Geometry: final body of the model. Coordinates: model frame, mm. A direction names the side the tool comes from. Give positions to 0.01 mm unless a question says otherwise; leave off trailing zeros. Write each loop counter-clockwise with the first axis right and the second up, starting at its lowest first coordinate (ties: lowest second). Pieces come first, ordered by that corner, then holes.
from build123d import *

# Parameters (mm, degrees)
SKETCH1_R                = 2.1
BOSS_EXTRUDE1_DEPTH      = 40
BOSS_EXTRUDE3_DEPTH      = 14
BOSS_EXTRUDE3_DEPTH_BACK = 14
SKETCH2_R                = 2.1


with BuildPart() as part:
    # Sketch1 → Boss-Extrude1 (new body)
    with BuildSketch(Plane(origin=(0, 0, 0), x_dir=(1, 0, 0), z_dir=(0, 1, 0))):
        Polygon((5, 0), (2.5, 4.330127019), (-2.5, 4.330127019), (-5, 0), (-2.5, -4.330127019), (2.5, -4.330127019), align=None)
        with Locations(Location((0, 0, 0), (0, 0, 270))):
            Circle(SKETCH1_R, mode=Mode.SUBTRACT)
    extrude(amount=BOSS_EXTRUDE1_DEPTH)

    # Sketch2 → Boss-Extrude3 (add, two sides: drawn at the far end of the back side and taken through both)
    with BuildSketch(Plane(origin=(0, 20, 0), x_dir=(1, 0, 0), z_dir=(0, 1, 0)).offset(-BOSS_EXTRUDE3_DEPTH_BACK)):
        with Locations(Location((0, 0, 0), (0, 0, 270))):
            Circle(SKETCH2_R)
    extrude(amount=BOSS_EXTRUDE3_DEPTH + BOSS_EXTRUDE3_DEPTH_BACK)


solid = part.part
Q1. Section C-C on z = -0.5. Output: boundary loops of the cut face in (x, y), plus the area to 3 significant figures.
Filled sheet:
outline: (-4.71, 0) - (-2.04, 0) - (-2.04, 6) - (2.04, 6) - (2.04, 0) - (4.71, 0) - (4.71, 40) - (2.04, 40) - (2.04, 34) - (-2.04, 34) - (-2.04, 40) - (-4.71, 40) - close
area: 328 mm2
Q2. Ray query, line 1 along Y through (x, z) = (0, 0.75); line 2 along X through (y, z) = (9.5, -3.75); line 3 along X through (y, z) = (7.5, -1.5). Return the intervals inside material, ascending.
Filled sheet:
line 1: y = 6 to 34
line 2: x = -2.83 to 2.83
line 3: x = -4.13 to 4.13
Q3. Access query for faces 1 (the cylindrical face through (0.631, 36.958, 2.003)), 2 (the flat face through (2.2, 40, -1)), 3 (the cylindrical face through (0.631, 2.958, 2.003)). Directions: +Z, -Z, +X, -X, +Y, -Y. A direction counts if a zero-diameter tool reaches every point of the face in a straight line with its end or side. Return the directions, or none.
Filled sheet:
face 1: +Y
face 2: +Z, -Z, +X, -X, +Y
face 3: -Y
Q4. Section D-D on y = 19.5. Output: boundary loops of the cut face in (x, z), plus the area to 3 significant figures.
Filled sheet:
outline: (-5, 0) - (-2.5, -4.33) - (2.5, -4.33) - (5, 0) - (2.5, 4.33) - (-2.5, 4.33) - close
area: 65.0 mm2
Q5. Section B-B on x = 0. Output: boundary loops of the cut face in (y, z).
Filled sheet:
outline: (0, -4.33) - (40, -4.33) - (40, -2.1) - (34, -2.1) - (34, 2.1) - (40, 2.1) - (40, 4.33) - (0, 4.33) - (0, 2.1) - (6, 2.1) - (6, -2.1) - (0, -2.1) - close
Q6. Pull-direction query (Z, two-part tool) for faces 4 (the flat face through (0, 6, 0)), 5 (the flat face through (0, 34, 0)), 6 (the flat face through (-3.77, 19.72, 2.13)), 7 (the flat face through (0, 20, -4.33)); classes: released by +Z, released by -Z, zero draft, split by the parting line, or undercut.
Filled sheet:
face 4: undercut
face 5: undercut
face 6: released by +Z
face 7: released by -Z
Q7. Section A-A on y = 36. Output: boundary loops of the cut face in (x, z).
Filled sheet:
outline: (-5, 0) - (-2.5, -4.33) - (2.5, -4.33) - (5, 0) - (2.5, 4.33) - (-2.5, 4.33) - close; hole circle Ø4.2 at (0, 0)
Q8. Pin query (flat end, axial travel): P1, Ø2, axis at x = -4, y = 21, coming from the -Z side; P2, Ø2, axis at x = -1, z = 0, coming from the -Y side; P3, Ø2, axis at x = 0, z = 0, coming from the +Y side. Return the tip coordinate at first contact, or that it passes through.
Filled sheet:
P1: stops at z = -3.46
P2: stops at y = 6
P3: stops at y = 34
